The drawing under review shows one solid part. Ordinate dimensions are in mm from its lowest x, y, z. A direction names the side the tool comes from. Coordinates: 2 decimals unless noted, no trailing zeros. Order: outer loops, then holes, each group sorted by start corner. A loop starts at its lowest first (then second) coordinate and runs counter-clockwise, first axis right, second up. Notation, with made-up numbers: (-34.5, 37) - (-7.5, 37) arc R23 ccw to (-7.5, 60) - close; hole circle Ø2 at (-24, 2.5). An arc over 180 degrees is marked (long way). Answer in a Markdown table with one row per item.
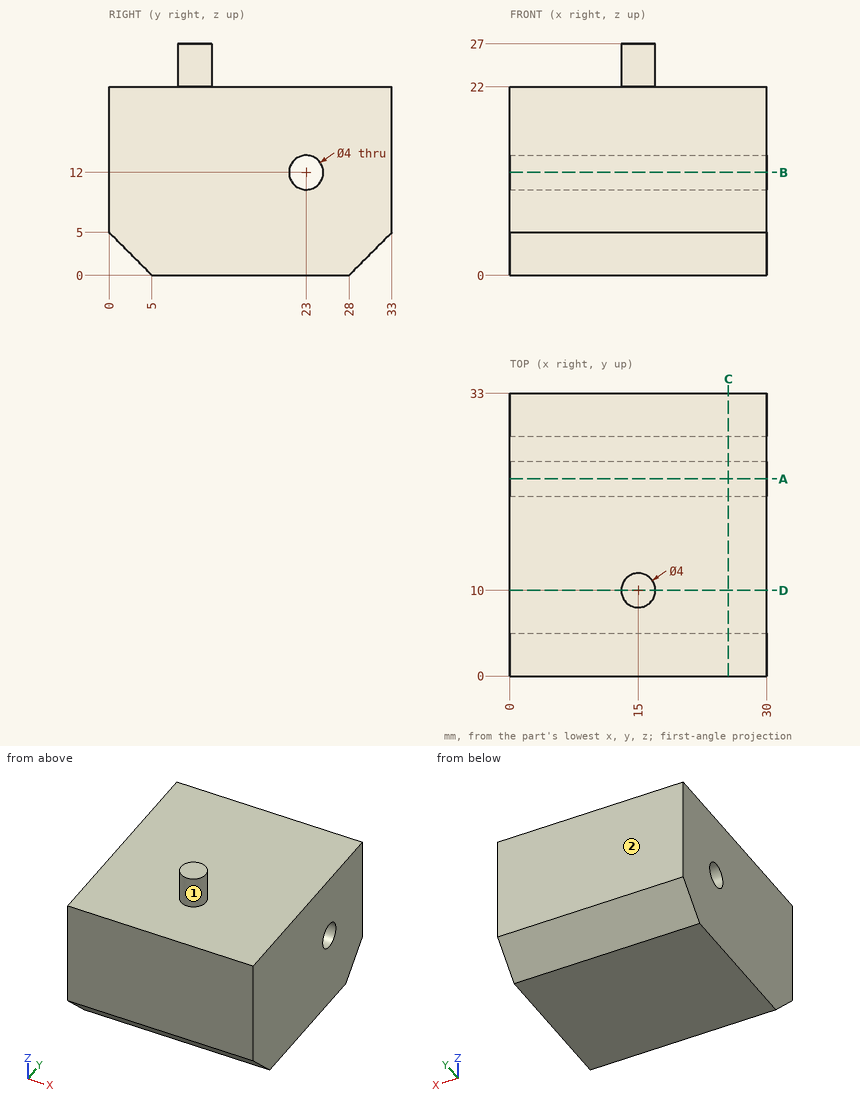
Item 1: To check wall thickness, follow line 1 (Z direction, x = 19.75, y = 23); line 2 (Z direction, x = 28.25, y = 15); line 3 (Y direction, x = 4.75, z = 11.75). State the ranges of each line that lie inside material, in increasing order. Write a range as from..to.
Check values:
| item | result |
|---|---|
| line 1 | 0..10, 14..22 |
| line 2 | 0..22 |
| line 3 | 0..21.02, 24.98..33 |
Item 2: We need section D-D, the plane y = 10. Write out the cut boundary in (x, z).
Check values:
| item | result |
|---|---|
| outline | (0, 0) - (30, 0) - (30, 22) - (17, 22) - (17, 27) - (13, 27) - (13, 22) - (0, 22) - close |
Item 3: We need section B-B, the plane z = 12. Write out the cut boundary in (x, y).
Check values:
| item | result |
|---|---|
| outline | (0, 0) - (30, 0) - (30, 21) - (0, 21) - close; (0, 25) - (30, 25) - (30, 33) - (0, 33) - close |
Item 4: We need section C-C, the plane x = 25.5. Write out the cut boundary in (y, z).
Check values:
| item | result |
|---|---|
| outline | (0, 5) - (5, 0) - (28, 0) - (33, 5) - (33, 22) - (0, 22) - close; hole circle Ø4 at (23, 12) |
Item 5: Clearance check with a flat-ended pin moving along its axis: pin 1 Ø1.5 at (x, y) = (5.5, 25) entering from +Z. State where the tip first meets the part, or that it passes through.
Check values:
| item | result |
|---|---|
| pin 1 | z = 22 |
Item 6: We need section A-A, the plane y = 23. Write out the cut boundary in (x, z), then the cut area to 3 significant figures.
Check values:
| item | result |
|---|---|
| outline | (0, 0) - (30, 0) - (30, 10) - (0, 10) - close; (0, 14) - (30, 14) - (30, 22) - (0, 22) - close |
| area | 540 mm^2 |
Item 7: Tool access review of the marked faces 1 and 2: name each direction out of +Z, -Z, +X, -X, +Y, -Y from which nothing blocks a thin tool from reaching the whole face with its end or side.
Check values:
| item | result |
|---|---|
| face 1 | +Z |
| face 2 | +Z, -Z, +X, -X, +Y |
